```python
from build123d import *

# Parameters (mm, degrees)
SKETCH1_W           = 35
SKETCH1_H           = 30
BOSS_EXTRUDE1_DEPTH = 28
SKETCH2_R           = 10
SKETCH2_R_2         = 4
CUT_EXTRUDE1_DEPTH  = 4
SKETCH4_R           = 4.2
CUT_EXTRUDE2_DEPTH  = 48


with BuildPart() as part:
    # Sketch1 → Boss-Extrude1 (new body)
    with BuildSketch(Plane(origin=(0, 0, 0), x_dir=(1, 0, 0), z_dir=(0, 1, 0))):
        with Locations((-2.651515152, -4.217171717)):
            Rectangle(SKETCH1_W, SKETCH1_H)
    extrude(amount=BOSS_EXTRUDE1_DEPTH)

    # Sketch2 → Cut-Extrude1 (cut)
    with BuildSketch(Plane.XY.offset(19.217171717)):
        with Locations((-2.538807386, 13.733372101)):
            Circle(SKETCH2_R)
        with Locations((-2.538807386, 13.733372101)):
            Circle(SKETCH2_R_2, mode=Mode.SUBTRACT)
    extrude(amount=-CUT_EXTRUDE1_DEPTH, mode=Mode.SUBTRACT)

    # Sketch4 → Cut-Extrude2 (cut)
    with BuildSketch(Plane.XY.offset(19.217171717)):
        with Locations((-2.597602696, 13.723084653)):
            Circle(SKETCH4_R)
    extrude(amount=-CUT_EXTRUDE2_DEPTH, mode=Mode.SUBTRACT)


solid = part.part
```
For this review, take the finished solid that the model builds, in its own axes (mm). A direction names the side the tool comes from. Give positions to 0.01 mm unless a question says otherwise; leave off trailing zeros. Write each loop counter-clockwise with the first axis right and the second up, starting at its lowest first coordinate (ties: lowest second). Pieces come first, ordered by that corner, then holes. Notation, with made-up numbers: M -35,-40 L -4,-40 A30 ccw -4,-13 Z; hole C 58,65.5 d8. An arc over 180 degrees is marked long. One line per item, written item: value.
1) For faces 4 (the cylindrical face through (-3.144, 17.887, 2.399)), 5 (the flat face through (2, 14, 15.217)), list the 3-axis set-ups (+Z, -Z, +X, -X, +Y, -Y) from which the entire face can be reached by the end or side of a thin tool; tool diameter is ignored.
Results are:
face 4: +Z, -Z
face 5: +Z
2) The part is to be moulded in two halves that separate along Y. For faces 1 (the cylindrical face through (-3.84, 23.65, 17.25)), 2 (the flat face through (-3, 28, 4)), 3 (the flat face through (-11, 20, 19.217)), say which applies: +Y half, -Y half, draft (parallel to the pull), parting line (faces both ways), or undercut.
Results are:
face 1: undercut
face 2: +Y half
face 3: draft
3) Take a section at A-A, the plane x = 1. Write out the cut boundary in (y, z), then the cut area to 3 significant figures.
Results are:
outline: M 0,-10.78 L 11.56,-10.78 L 11.56,15.22 L 4.38,15.22 L 4.38,19.22 L 0,19.22 Z; M 15.89,-10.78 L 28,-10.78 L 28,19.22 L 23.09,19.22 L 23.09,15.22 L 15.89,15.22 Z
area: 652 mm²
4) Take a section at B-B, the plane y = 12.75. Write out the cut boundary in (x, z), then the cut area to 3 significant figures.
Results are:
outline: M -20.15,-10.78 L -6.68,-10.78 L -6.68,15.22 L -12.49,15.22 L -12.49,19.22 L -20.15,19.22 Z; M 1.49,-10.78 L 14.85,-10.78 L 14.85,19.22 L 7.41,19.22 L 7.41,15.22 L 1.49,15.22 Z
area: 758 mm²
5) For line 1 (Y direction, x = -2.5, z = 2.25); line 2 (Z direction, x = 6, y = 11.75); line 3 (X direction, y = 11.75, z = 12.75), list the stretches that pass through material, from the lowest coordinate up. Write a range as from..to.
Results are:
line 1: y = 0..9.52, 17.92..28
line 2: z = -10.78..15.22
line 3: x = -20.15..-6.31, 1.11..14.85
6) For P1, Ø1.5, axis at x = -2, y = 21, coming from the +Z side, flat-tipped, find the tip position at first contact; note if it passes through.
Results are:
P1: stops at z = 15.22
7) Take a section at D-D, the plane y = 20.5. Write out the cut boundary in (x, z), then the cut area to 3 significant figures.
Results are:
outline: M -20.15,-10.78 L 14.85,-10.78 L 14.85,19.22 L 4.82,19.22 L 4.82,15.22 L -9.9,15.22 L -9.9,19.22 L -20.15,19.22 Z
area: 991 mm²
8) Take a section at C-C, the plane z = 3. Write out the cut boundary in (x, y), then the cut area to 3 significant figures.
Results are:
outline: M -20.15,0 L 14.85,0 L 14.85,28 L -20.15,28 Z; hole C -2.6,13.72 d8.4
area: 925 mm²
